For this review, use the dimensioned drawing (mm, ordinates from the lowest corner) and the shaded views. A direction names the side the tool comes from. Coordinates: 2 decimals unless noted, no trailing zeros. Order: outer loops, then holes, each group sorted by start corner. A loop starts at its lowest first (then second) coordinate and runs counter-clockwise, first axis right, second up. Notation, with made-up numbers: M 82,62.25 L 112,62.25 A21 cw 112,74.25 Z; hole C 16.25,89.25 d4. An arc over 180 degrees is marked long. Answer in a Markdown table with one row per item.
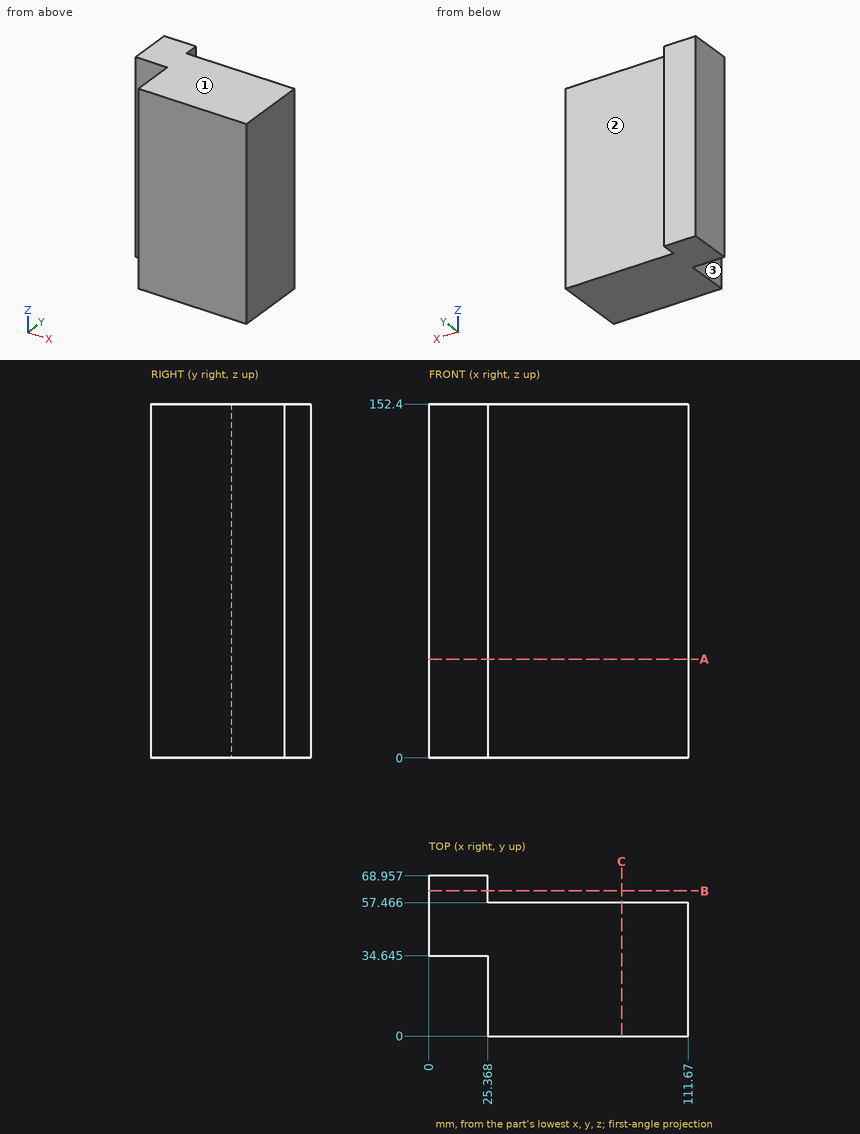
(1) For the marked faces 1, 2 and 3, list the 3-axis set-ups (+Z, -Z, +X, -X, +Y, -Y) from which the entire face can be reached by the end or side of a thin tool; tool diameter is ignored.
Return value:
| item | result |
|---|---|
| face 1 | +Z, +X, -X, +Y, -Y |
| face 2 | +Z, -Z, +X, +Y |
| face 3 | +Z, -Z, -X, -Y |
(2) Add section C-C, the plane x = 83. Give the boundary of the cut face in (y, z) (1 decimal), and give its area (3 significant figures).
Return value:
| item | result |
|---|---|
| outline | M 0,0 L 57.5,0 L 57.5,152.4 L 0,152.4 Z |
| area | 8,760 mm2 |
(3) Add section B-B, the plane y = 62.5. Give the boundary of the cut face in (x, z).
Return value:
| item | result |
|---|---|
| outline | M 0,0 L 25.37,0 L 25.37,152.4 L 0,152.4 Z |
(4) Insertion check: pin 1 Ø10 at (x, z) = (54, 92.5) entering from +Y; pin 2 Ø6 at (y, z) = (61, 106.5) entering from +X; pin 3 Ø12 at (x, y) = (16.5, 11) entering from +Z. Each pin has a flat end and moves straight along its axis. Give the tip position at first contact, or say it passes through.
Return value:
| item | result |
|---|---|
| pin 1 | stops at y = 57.47 |
| pin 2 | stops at x = 25.37 |
| pin 3 | passes through |
(5) Add section A-A, the plane z = 42.5. Give the boundary of the cut face in (x, y) (1 decimal), and give its area (3 significant figures).
Return value:
| item | result |
|---|---|
| outline | M 0,34.6 L 25.4,34.6 L 25.4,0 L 111.7,0 L 111.7,57.5 L 25.4,57.5 L 25.4,69 L 0,69 Z |
| area | 5,830 mm2 |
(6) For line 1 along X through (y, z) = (66.5, 31); line 2 along Y through (x, z) = (17.5, 85) (1 decimal); line 3 along Y through (x, z) = (48, 91) (1 decimal), list the stretches that pass through material, from the lowest coordinate up. Write a range as from..to.
Return value:
| item | result |
|---|---|
| line 1 | x = 0..25.37 |
| line 2 | y = 34.6..69 |
| line 3 | y = 0..57.5 |
